Part model, mm, in its own coordinate system. Face numbers are marked on the shaded views. A direction names the side the tool comes from. Give positions to 0.01 mm unless a question says otherwise; leave off trailing zeros. Order: outer loops, then holes, each group sorted by start corner. A loop starts at its lowest first (then second) coordinate and runs counter-clockwise, first axis right, second up. Notation, with made-up numbers: (87, -26.5) - (112, -26.5) arc R24 cw to (112, -15.5) - close; hole circle Ø2 at (-23.5, 26.5). An arc over 180 degrees is marked (long way). Use a Markdown table: item, result. Add a question column.
from build123d import *
from build123d.topology import SkipClean

# Parameters (mm, degrees)
SKETCH2_R                 = 9.5
BOSS_EXTRUDE1_DEPTH       = 5
SKETCH3_W                 = 35
SKETCH3_H                 = 85.128
BOSS_EXTRUDE2_DEPTH       = 3
BOSS_EXTRUDE3_START       = 5
SKETCH4_R                 = 13
SKETCH4_R_2               = 9.5
BOSS_EXTRUDE3_DEPTH       = 5
SKETCH5_W                 = 35
SKETCH5_H                 = 9
BOSS_EXTRUDE4_DEPTH       = 3
M3X0_5_TAPPED_HOLE1_D     = 2.5
M3X0_5_TAPPED_HOLE1_DEPTH = 3
BOSS_EXTRUDE5_DEPTH       = 24
SKETCH11_R                = 9.652
CUT_EXTRUDE1_DEPTH        = 14
CUT_EXTRUDE2_START        = -5
CUT_EXTRUDE2_DEPTH        = 5
CUT_EXTRUDE4_DEPTH        = 3
SKETCH15_W                = 35
SKETCH15_H                = 25.028
CUT_EXTRUDE5_DEPTH        = 12
M3X0_5_TAPPED_HOLE2_D     = 2.5
M3X0_5_TAPPED_HOLE2_DEPTH = 6.5
M3X0_5_TAPPED_HOLE2_TIP   = 0.751075774
FILLET7_R                 = 7
BOSS_EXTRUDE6_START       = -5
BOSS_EXTRUDE6_DEPTH       = 5
FILLET3_R                 = 5
CUT_EXTRUDE6_START        = -25
CUT_EXTRUDE6_DEPTH        = 25
FILLET5_R                 = 10
FILLET4_R                 = 3
M4X0_7_TAPPED_HOLE1_D     = 3.3


with BuildPart() as part:
    # Sketch2 → Boss-Extrude1 (new body)
    with BuildSketch(Plane.XY):
        with BuildLine():
            Line((-18.994017858, 0.476744791), (-17.5, 60))
            Line((-17.5, 60), (17.5, 60))
            Line((17.5, 60), (18.994017858, 0.476744791))
            ThreePointArc((18.994017858, 0.476744791), (0, -19), (-18.994017858, 0.476744791))
        make_face()
        Circle(SKETCH2_R, mode=Mode.SUBTRACT)
    extrude(amount=BOSS_EXTRUDE1_DEPTH)

    # Sketch3 → Boss-Extrude2 (add)
    with BuildSketch(Plane(origin=(0, 60, 0), x_dir=(1, 0, 0), z_dir=(0, 1, 0))):
        with Locations((0, 37.564)):
            Rectangle(SKETCH3_W, SKETCH3_H)
    extrude(amount=BOSS_EXTRUDE2_DEPTH)

    # Sketch4 → Boss-Extrude3 (add)
    with SkipClean():  # the faces are left unmerged after this step: merging them gives an invalid solid
        with BuildSketch(Plane(origin=(0, 0, 0), x_dir=(-1, 0, 0), z_dir=(0, 0, -1)).offset(BOSS_EXTRUDE3_START)):
            with Locations(Location((0, 0, 0), (0, 0, 180))):
                Circle(SKETCH4_R)
            Circle(SKETCH4_R_2, mode=Mode.SUBTRACT)
        extrude(amount=-BOSS_EXTRUDE3_DEPTH)

    # Sketch5 → Boss-Extrude4 (add)
    with SkipClean():  # the faces are left unmerged after this step: merging them gives an invalid solid
        with BuildSketch(Plane(origin=(0, 0, -80.128), x_dir=(-1, 0, 0), z_dir=(0, 0, -1))):
            with Locations((0, 55.5)):
                Rectangle(SKETCH5_W, SKETCH5_H)
        extrude(amount=-BOSS_EXTRUDE4_DEPTH)

    # M3x0.5 Tapped Hole1
    with Locations(Plane(origin=(0, 0, -80.128), x_dir=(1, 0, 0), z_dir=(0, 0, -1))):
        with Locations((12, -55.5), (0, -55.5), (-12, -55.5)):
            Hole(M3X0_5_TAPPED_HOLE1_D / 2, depth=M3X0_5_TAPPED_HOLE1_DEPTH)

    # Sketch10 → Boss-Extrude5 (add)
    with SkipClean():  # the faces are left unmerged after this step: merging them gives an invalid solid
        with BuildSketch(Plane.XY.offset(5)):
            Polygon((-5, 85.612930278), (-5, 63), (17.5, 63), (17.5, 64), (9.633536704, 85.612930278), align=None)
        extrude(amount=-BOSS_EXTRUDE5_DEPTH)

    # Sketch11 → Cut-Extrude1 (cut)
    with SkipClean():  # the faces are left unmerged after this step: merging them gives an invalid solid
        with BuildSketch(Plane(origin=(-1.821352029, 117.084978414, 0), x_dir=(0, 0, -1), z_dir=(-0.9396926207859069, -0.34202014332567293, 0))):
            with Locations(Location((7.5, 44.49185408, 0), (0, 0, 90))):
                Circle(SKETCH11_R)
        extrude(amount=CUT_EXTRUDE1_DEPTH, mode=Mode.SUBTRACT)

    # Sketch12 → Cut-Extrude2 (cut)
    with SkipClean():  # the faces are left unmerged after this step: merging them gives an invalid solid
        with BuildSketch(Plane.XY.offset(5).offset(CUT_EXTRUDE2_START)):
            with BuildLine():
                Line((-13.548939673, 58), (13.548939673, 58))
                Line((13.548939673, 58), (14.702658736, 12.034609511))
                ThreePointArc((14.702658736, 12.034609511), (0, 19), (-14.702658736, 12.034609511))
                Line((-14.702658736, 12.034609511), (-13.548939673, 58))
            make_face()
        extrude(amount=CUT_EXTRUDE2_DEPTH, mode=Mode.SUBTRACT)

    # Sketch14 → Cut-Extrude4 (cut)
    with SkipClean():  # the faces are left unmerged after this step: merging them gives an invalid solid
        with BuildSketch(Plane(origin=(0, 63, 0), x_dir=(1, 0, 0), z_dir=(0, 1, 0))):
            with BuildLine():
                Line((-14.1, 51.5), (-14.1, 27.5))
                ThreePointArc((-14.1, 27.5), (-12.5, 25.9), (-10.9, 27.5))
                Line((-10.9, 27.5), (-10.9, 51.5))
                ThreePointArc((-10.9, 51.5), (-12.5, 53.1), (-14.1, 51.5))
            make_face()
            with BuildLine():
                Line((-1.6, 51.5), (-1.6, 27.5))
                ThreePointArc((-1.6, 27.5), (0, 25.9), (1.6, 27.5))
                Line((1.6, 27.5), (1.6, 51.5))
                ThreePointArc((1.6, 51.5), (0, 53.1), (-1.6, 51.5))
            make_face()
            with BuildLine():
                Line((10.9, 51.5), (10.9, 27.5))
                ThreePointArc((10.9, 27.5), (12.5, 25.9), (14.1, 27.5))
                Line((14.1, 27.5), (14.1, 51.5))
                ThreePointArc((14.1, 51.5), (12.5, 53.1), (10.9, 51.5))
            make_face()
            with BuildLine():
                Line((-7.85, 51.5), (-7.85, 27.5))
                ThreePointArc((-7.85, 27.5), (-6.25, 25.9), (-4.65, 27.5))
                Line((-4.65, 27.5), (-4.65, 51.5))
                ThreePointArc((-4.65, 51.5), (-6.25, 53.1), (-7.85, 51.5))
            make_face()
            with BuildLine():
                Line((4.65, 51.5), (4.65, 27.5))
                ThreePointArc((4.65, 27.5), (6.25, 25.9), (7.85, 27.5))
                Line((7.85, 27.5), (7.85, 51.5))
                ThreePointArc((7.85, 51.5), (6.25, 53.1), (4.65, 51.5))
            make_face()
        extrude(amount=-CUT_EXTRUDE4_DEPTH, mode=Mode.SUBTRACT)

    # Sketch15 → Cut-Extrude5 (cut)
    with SkipClean():  # the faces are left unmerged after this step: merging them gives an invalid solid
        with BuildSketch(Plane(origin=(0, 63, 0), x_dir=(1, 0, 0), z_dir=(0, 1, 0))):
            with Locations((0, 67.614)):
                Rectangle(SKETCH15_W, SKETCH15_H)
        extrude(amount=-CUT_EXTRUDE5_DEPTH, mode=Mode.SUBTRACT)

    # M3x0.5 Tapped Hole2
    with Locations(Plane.XY.offset(5)):
        with Locations((0, 15), (15, 0), (0, -15), (-15, 0)):
            Hole(M3X0_5_TAPPED_HOLE2_D / 2, depth=M3X0_5_TAPPED_HOLE2_DEPTH)
            with Locations((0, 0, -(M3X0_5_TAPPED_HOLE2_DEPTH + M3X0_5_TAPPED_HOLE2_TIP / 2))):  # 118° drill point
                Cone(0, M3X0_5_TAPPED_HOLE2_D / 2, M3X0_5_TAPPED_HOLE2_TIP, mode=Mode.SUBTRACT)

    # Fillet7
    fillet7_edges = [part.edges().sort_by_distance(p)[0] for p in [
        (2.316768352, 85.612930278, 5),
        (2.316768352, 85.612930278, -19),
    ]]
    fillet(fillet7_edges, radius=FILLET7_R)

    # Sketch22 → Boss-Extrude6 (add)
    with SkipClean():  # the faces are left unmerged after this step: merging them gives an invalid solid
        with BuildSketch(Plane.XY.offset(5).offset(BOSS_EXTRUDE6_START)):
            with BuildLine():
                Line((-5, 58), (-5, 18.33030278))
                ThreePointArc((-5, 18.33030278), (5.783107735, 18.098498969), (14.702658736, 12.034609511))
                Line((14.702658736, 12.034609511), (13.548939673, 58))
                Line((13.548939673, 58), (-5, 58))
            make_face()
        extrude(amount=BOSS_EXTRUDE6_DEPTH)

    # Fillet3
    # the kernel refuses this fillet: 5 mm, written as the material it adds along each edge
    with BuildSketch(Plane(origin=(-5, 63, -19), x_dir=(0, 1, 0), z_dir=(1, 0, 0))) as fillet3_piece_1_section:
        with BuildLine():
            CenterArc((FILLET3_R, -FILLET3_R), FILLET3_R, 90, 90)
            Line((0, -FILLET3_R), (0, 0))
            Line((0, 0), (FILLET3_R, 0))
        make_face()
    fillet3_piece_1 = extrude(amount=22.5, mode=Mode.PRIVATE)
    fillet3_piece_1 = split(fillet3_piece_1, bisect_by=Plane(origin=(16.135828419, 67.748030616, -20.138902613), z_dir=(-0.9396926207859069, -0.34202014332567293, 0)), keep=Keep.TOP, mode=Mode.PRIVATE)
    add(fillet3_piece_1)

    # Sketch25 → Cut-Extrude6 (cut)
    with SkipClean():  # the faces are left unmerged after this step: merging them gives an invalid solid
        with BuildSketch(Plane.XY.offset(5).offset(CUT_EXTRUDE6_START)):
            with BuildLine():
                Line((-5, 63), (-17.5, 63))
                Line((-17.5, 63), (-18.994017858, 0.476744791))
                ThreePointArc((-18.994017858, 0.476744791), (-14.953782346, 11.721108887), (-5, 18.33030278))
                Line((-5, 18.33030278), (-5, 63))
            make_face()
        extrude(amount=CUT_EXTRUDE6_DEPTH, mode=Mode.SUBTRACT)

    # Fillet5
    # the kernel refuses this fillet: 10 mm, written as the material it adds along each edge
    with BuildSketch(Plane(origin=(-5, 60, 0), x_dir=(0, 0, -1), z_dir=(1, 0, 0))) as fillet5_piece_1:
        with BuildLine():
            CenterArc((FILLET5_R, -FILLET5_R), FILLET5_R, 90, 90)
            Line((0, -FILLET5_R), (0, 0))
            Line((0, 0), (FILLET5_R, 0))
        make_face()
    extrude(amount=22.5)
    with BuildSketch(Plane(origin=(-5, 60, 0), x_dir=(0, 0, -1), z_dir=(1, 0, 0))) as fillet5_piece_2_section:
        with BuildLine():
            CenterArc((FILLET5_R, -FILLET5_R), FILLET5_R, 90, 90)
            Line((0, -FILLET5_R), (0, 0))
            Line((0, 0), (FILLET5_R, 0))
        make_face()
    fillet5_piece_2 = extrude(amount=47.5, mode=Mode.PRIVATE)
    fillet5_piece_2 = split(fillet5_piece_2, bisect_by=Plane(origin=(17.5, 55.698819483, -1.064725127), z_dir=(1, 0, 0)), keep=Keep.TOP, mode=Mode.PRIVATE)
    fillet5_piece_2 = split(fillet5_piece_2, bisect_by=Plane(origin=(17.607924501, 55.700173495, -1.064725127), z_dir=(-0.9996851504403609, -0.0250918311215615, 0)), keep=Keep.TOP, mode=Mode.PRIVATE)
    add(fillet5_piece_2)

    # Fillet4
    fillet4_edges = [part.edges().sort_by_distance(p)[0] for p in [
        (-5, 18.33030278, 2.5),
        (-17.5, 61.5, -20),
        (-5, 61.5, -20),
    ]]
    fillet(fillet4_edges, radius=FILLET4_R)

    # M4x0.7 Tapped Hole1 (through all)
    with Locations(Plane.XY.offset(5)):
        with Locations((0, 34)):
            Hole(M4X0_7_TAPPED_HOLE1_D / 2)


solid = part.part
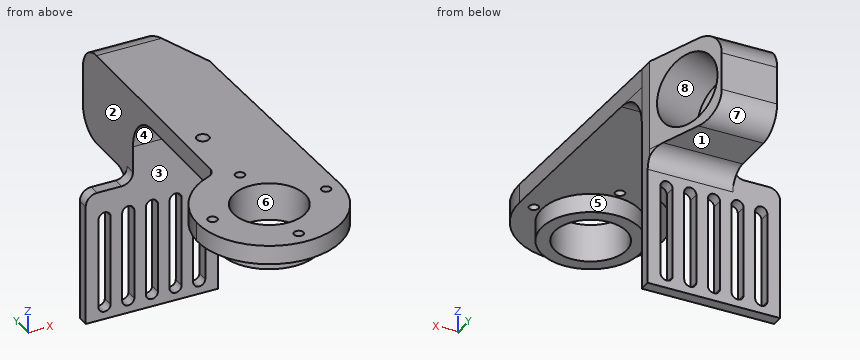
1. Pin check, flat tips, straight feed: P1, Ø0.9, axis at y = 61, z = -40.5, coming from the -X side; P2, Ø2.5, axis at y = 61, z = -42, coming from the +X side; P3, Ø3, axis at x = -6.5, z = -44, coming from the +Y side. Stop position of each tip, or through.
2. Tool access for the marked faces 1, 2, 3 and 4: list every direction of +Z, -Z, +X, -X, +Y, -Y with a clear straight run to the whole face (end or side of a thin tool).
3. Cut at A-A (z = -44). Write the cut outline in (x, y).
4. Cut at B-B (y = 34). Write the cut outline in (x, z), plus the area to 3 significant figures.
5. Mould opens along X. For the marked faces 5, 6, 7 and 8 say: released by +X, released by -X, zero draft, split by the parting line, or undercut.
6. Drill centre lines: probe 1 along X at (y, z) = (62, -46); probe 2 along Y at (x, z) = (0, 2.75); probe 3 along Z at (x, y) = (-3, 21). Where is each one in solid material? Low to high. Write a range as [from, to].
7. Cut at C-C (x = 0). State how many separate pieces and enclosed holes the cut face has, plus the area to 3 significant figures.
8. Cut at D-D (y = 54.5). Write the cut outline in (x, z), plus the area to 3 significant figures.
Responses:
| question | item | result |
|---|---|---|
| 1 | P1 | stops at x = -17.5 |
| 1 | P2 | stops at x = 17.5 |
| 1 | P3 | stops at y = 63 |
| 2 | face 1 | -Z, +X, -X, +Y |
| 2 | face 2 | +Z, -X, +Y |
| 2 | face 3 | -Z, +X, -X, -Y |
| 2 | face 4 | -Z, +X, -X |
| 3 | outline | (-17.5, 60) - (-14.1, 60) - (-14.1, 63) - (-17.5, 63) - close; (-10.9, 60) - (-7.85, 60) - (-7.85, 63) - (-10.9, 63) - close; (-4.65, 60) - (-1.6, 60) - (-1.6, 63) - (-4.65, 63) - close; (1.6, 60) - (4.65, 60) - (4.65, 63) - (1.6, 63) - close; (7.85, 60) - (10.9, 60) - (10.9, 63) - (7.85, 63) - close; (14.1, 60) - (17.5, 60) - (17.5, 63) - (14.1, 63) - close |
| 4 | outline | (-5, 0) - (-1.65, 0) - (-1.65, 5) - (-5, 5) - close; (1.65, 0) - (18.15, 0) - (18.15, 5) - (1.65, 5) - close |
| 4 | area | 99.3 mm² |
| 5 | face 5 | split by the parting line |
| 5 | face 6 | undercut |
| 5 | face 7 | zero draft |
| 5 | face 8 | undercut |
| 6 | probe 1 | x = [-17.5, -14.1], [-10.9, -7.85], [-4.65, -1.6], [1.6, 4.65], [7.85, 10.9], [14.1, 17.5] |
| 6 | probe 2 | y = [-19, -16.25], [-13.75, -9.5], [9.5, 13.75], [16.25, 32.35], [35.65, 83.75] |
| 6 | probe 3 | z = [0, 5] |
| 7 | separate pieces | 6 |
| 7 | enclosed holes | 1 |
| 7 | area | 799 mm² |
| 8 | outline | (-5, -1.07) - (17.64, -1.07) - (17.64, 5) - (-5, 5) - close |
| 8 | area | 137 mm² |
